Could you check a few things on this model? Use its own coordinates, in mm. A direction names the side the tool comes from. Round coordinates to 2 decimals unless told otherwise and drop trailing zeros. Loops run counter-clockwise (first coordinate to the right, second up) from the corner with the lowest first, then second, coordinate; pieces in that order, holes last. Notation, with made-up numbers: M 42.5,1 L 52.5,1 A32 cw 52.5,39 Z; hole C 44.25,43 d2. An arc over 180 degrees is marked long. One line per item, written item: value. Start each with the question number.
Q1. Imagine slicing it at B-B (y = 0). Please give me the cut outline in (x, z).
Q2. I'm going to push flat-ended pins straight in: pin 1 Ø1.5 at (x, z) = (-1.5, 19) entering from +Y; pin 2 Ø3 at (x, z) = (-0.5, -14) entering from -Y; pin 3 Ø2 at (x, y) = (2, 3) entering from +Z; pin 4 Ø1.6 at (x, z) = (0, -13) entering from -Y. Where does each tip first touch, or does it pass through?
Q3. Thinking about a two-plate mould opening in Z: for faces 6 (the face through (0, 0, -12)), 7 (the face through (0, -2, -10)), 8 (the face through (-1, 1.5, 38)), 9 (the face through (0, 0, -16)), which applies, released by +Z, released by -Z, zero draft, split by the parting line, or undercut?
Q4. Imagine slicing it at D-D (z = 39). Please give me the cut outline in (x, y), then the cut area to 3 significant figures.
Q5. Imagine slicing it at A-A (z = -13). Please give me the cut outline in (x, y), then the cut area to 3 significant figures.
Q6. Please list where these lines run through material, in increasing order: line 1 along X through (y, z) = (-0.65, 39); line 2 along Z through (x, y) = (-0.75, -0.5); line 3 along Z through (x, y) = (-0.5, -0.5).
Q7. Which directions (+Z, -Z, +X, -X, +Y, -Y) give clear straight access to the entire face, cutting with the end or side of a thin tool? Please do faces 1 (the face through (-1, -1.5, 38)), 2 (the face through (0.54, -2.44, -5.94)), 3 (the face through (1, -1.5, -14)), 4 (the face through (0, 2, -10)), 5 (the face through (-4.77, 0, 38)).
Q8. Imagine slicing it at C-C (x = 0). Please give me the cut outline in (y, z).
from build123d import *

# Parameters (mm, degrees)
SKETCH1_R           = 5
BOSS_EXTRUDE1_DEPTH = 35
SKETCH2_W           = 9.539392014
SKETCH2_H           = 3
BOSS_EXTRUDE2_DEPTH = 8
SKETCH3_R           = 2.5
BOSS_EXTRUDE3_DEPTH = 10
SKETCH4_W           = 4
SKETCH4_H           = 3
BOSS_EXTRUDE4_DEPTH = 3
SKETCH5_R           = 3
BOSS_EXTRUDE5_DEPTH = 3
FILLET1_R           = 2
FILLET4_R           = 2
SKETCH6_R           = 1
CUT_EXTRUDE1_DEPTH  = 44.774992861
SKETCH7_R           = 1
CUT_EXTRUDE2_DEPTH  = 44.774992861


with BuildPart() as part:
    # Sketch1 → Boss-Extrude1 (new body)
    with BuildSketch(Plane.XY):
        Circle(SKETCH1_R)
    extrude(amount=BOSS_EXTRUDE1_DEPTH)

    # Sketch2 → Boss-Extrude2 (add)
    with BuildSketch(Plane.XY.offset(35)):
        Rectangle(SKETCH2_W, SKETCH2_H)
    extrude(amount=BOSS_EXTRUDE2_DEPTH)

    # Sketch3 → Boss-Extrude3 (add)
    with BuildSketch(Plane(origin=(0, 0, 0), x_dir=(-1, 0, 0), z_dir=(0, 0, -1))):
        Circle(SKETCH3_R)
    extrude(amount=BOSS_EXTRUDE3_DEPTH)

    # Sketch4 → Boss-Extrude4 (add)
    with BuildSketch(Plane(origin=(0, 0, -10), x_dir=(-1, 0, 0), z_dir=(0, 0, -1))):
        Rectangle(SKETCH4_W, SKETCH4_H)
    extrude(amount=BOSS_EXTRUDE4_DEPTH)

    # Sketch5 → Boss-Extrude5 (add)
    with BuildSketch(Plane(origin=(0, -1.5, 0), x_dir=(-1, 0, 0), z_dir=(0, -1, 0))):
        with Locations((0, 13)):
            Circle(SKETCH5_R)
    extrude(amount=-BOSS_EXTRUDE5_DEPTH)

    # Fillet1
    fillet1_edges = [part.edges().sort_by_distance(p)[0] for p in [
        (4.769696007, 0, 43),
        (-4.769696007, 0, 43),
    ]]
    fillet(fillet1_edges, radius=FILLET1_R)

    # Fillet4
    fillet4_edges = [part.edges().sort_by_distance(p)[0] for p in [
        (2.5, 0, 0),
    ]]
    fillet(fillet4_edges, radius=FILLET4_R)

    # Sketch6 → Cut-Extrude1 (cut, through all)
    with BuildSketch(Plane(origin=(0, 1.5, 0), x_dir=(1, 0, 0), z_dir=(0, 1, 0))):
        with Locations(Location((0, 13, 0), (0, 0, 270))):
            Circle(SKETCH6_R)
    extrude(amount=-CUT_EXTRUDE1_DEPTH, mode=Mode.SUBTRACT)

    # Sketch7 → Cut-Extrude2 (cut, through all)
    with BuildSketch(Plane(origin=(0, 1.5, 0), x_dir=(1, 0, 0), z_dir=(0, 1, 0))):
        with Locations(Location((0, -39, 0), (0, 0, 270))):
            Circle(SKETCH7_R)
    extrude(amount=-CUT_EXTRUDE2_DEPTH, mode=Mode.SUBTRACT)


solid = part.part
Report:
1. outline: M -5,0 L -4.5,0 A2 cw -2.5,-2 L -2.5,-10 L -2,-10 L -2,-10.76 A3 ccw long 2,-10.76 L 2,-10 L 2.5,-10 L 2.5,-2 A2 cw 4.5,0 L 5,0 L 5,35 L 4.77,35 L 4.77,41 A2 ccw 2.77,43 L -2.77,43 A2 ccw -4.77,41 L -4.77,35 L -5,35 Z; hole C 0,-13 d2; hole C 0,39 d2
2. pin 1: stops at y = 4.94
2. pin 2: stops at y = -1.5
2. pin 3: stops at z = 35
2. pin 4: passes through
3. face 6: undercut
3. face 7: released by -Z
3. face 8: zero draft
3. face 9: undercut
4. outline: M -4.77,-1.5 L -1,-1.5 L -1,1.5 L -4.77,1.5 Z; M 1,-1.5 L 4.77,-1.5 L 4.77,1.5 L 1,1.5 Z
4. area: 22.6 mm²
5. outline: M -3,-1.5 L -1,-1.5 L -1,1.5 L -3,1.5 Z; M 1,-1.5 L 3,-1.5 L 3,1.5 L 1,1.5 Z
5. area: 12.0 mm²
6. line 1: x = -4.77 to -1, 1 to 4.77
6. line 2: z = -15.9 to -13.66, -12.34 to 38.34, 39.66 to 43
6. line 3: z = -15.96 to -13.87, -12.13 to 38.13, 39.87 to 43
7. face 1: +Z, +X, -X, -Y
7. face 2: none
7. face 3: -Z, +X, -X, -Y
7. face 4: -Z, +X, -X, +Y
7. face 5: +Z, -X, +Y, -Y
8. outline: M -5,0 L -4.5,0 A2 cw -2.5,-2 L -2.5,-10 L -1.5,-10 L -1.5,-12 L 1.5,-12 L 1.5,-10 L 2.5,-10 L 2.5,-2 A2 cw 4.5,0 L 5,0 L 5,35 L 1.5,35 L 1.5,38 L -1.5,38 L -1.5,35 L -5,35 Z; M -1.5,-16 L 1.5,-16 L 1.5,-14 L -1.5,-14 Z; M -1.5,40 L 1.5,40 L 1.5,43 L -1.5,43 Z
